```python
from build123d import *

# Parameters (mm, degrees)
SKETCH_1_R          = 6
EXTRUDE_1_DEPTH     = 1
SKETCH_2_R          = 4.075
SKETCH_2_R_2        = 3
EXTRUDE_2_DEPTH     = 3
CUT_EXTRUDE_START   = -3
SKETCH_3_R          = 3
CUT_EXTRUDE_1_DEPTH = 3
CHAMFER_1_SIZE      = 0.5


with BuildPart() as part:
    # 草图1 → 凸台-拉伸1 (new body)
    with BuildSketch(Plane(origin=(0, 0, 0), x_dir=(1, 0, 0), z_dir=(0, 1, 0))):
        with Locations(Location((-0.138701754, 0.180249091, 0), (0, 0, 270))):
            Circle(SKETCH_1_R)
    extrude(amount=EXTRUDE_1_DEPTH)

    # 草图2 → 凸台-拉伸2 (add)
    with BuildSketch(Plane(origin=(0, 1, 0), x_dir=(1, 0, 0), z_dir=(0, 1, 0))):
        with Locations(Location((-0.138701754, 0.180249091, 0), (0, 0, 270))):
            Circle(SKETCH_2_R)
        with Locations(Location((-0.138701754, 0.180249091, 0), (0, 0, 270))):
            Circle(SKETCH_2_R_2, mode=Mode.SUBTRACT)
    extrude(amount=EXTRUDE_2_DEPTH)

    # 草图3 → 切除-拉伸1 (cut)
    with BuildSketch(Plane(origin=(0, 1, 0), x_dir=(1, 0, 0), z_dir=(0, 1, 0)).offset(CUT_EXTRUDE_START)):
        with Locations(Location((-0.138701754, 0.180249091, 0), (0, 0, 270))):
            Circle(SKETCH_3_R)
    extrude(amount=CUT_EXTRUDE_1_DEPTH, mode=Mode.SUBTRACT)

    # 倒角1
    chamfer_1_edges = [part.edges().sort_by_distance(p)[0] for p in [
        (-0.138701754, 4, -4.255249091),
    ]]
    chamfer(chamfer_1_edges, length=CHAMFER_1_SIZE)


solid = part.part
```
Source: CAD feature listing. Evaluate the final solid. Frame: model axes, mm. Give positions to 0.01 mm unless a question says otherwise; leave off trailing zeros. Loops run counter-clockwise (first coordinate to the right, second up) from the corner with the lowest first, then second, coordinate; pieces in that order, holes last. Notation, with made-up numbers: M -27,51.5 L -12,51.5 A22 cw -12,58.5 Z; hole C -17,0.25 d10. An arc over 180 degrees is marked long. Put each result on its own line as item: value.
Q1. Mould query, pull axis Z, two halves, no side actions, for faces 1 (the flat face through (-1, 1, 4)), 2 (the cylindrical face through (-2.618, 2.232, -3.414)), 3 (the cylindrical face through (-1.29, 1.97, 2.59)). Classes: released by +Z, released by -Z, zero draft, split by the parting line, or undercut.
Response values:
face 1: zero draft
face 2: split by the parting line
face 3: undercut
Q2. Section B-B (x = 5). Return the cut outline in (y, z).
Response values:
outline: M 0,-3.28 L 1,-3.28 L 1,2.92 L 0,2.92 Z
Q3. Section C-C (z = 4.25). Return the cut outline in (x, y).
Response values:
outline: M -4.19,0 L 3.91,0 L 3.91,1 L -4.19,1 Z
Q4. Line query: probe 1 along Z at (x, y) = (-1.25, 2.9); probe 2 along Y at (x, z) = (0.75, -3.75); probe 3 along Z at (x, y) = (1.75, 0.2). Output: solid intervals per line, ascending. Write a range as [from, to].
Response values:
probe 1: z = [-4.1, -2.97], [2.61, 3.74]
probe 2: y = [0, 3.9]
probe 3: z = [-5.88, -2.51], [2.15, 5.51]
Q5. Pin query (flat end, axial travel): P1, Ø3, axis at x = -3, z = 4.5, coming from the +Y side; P2, Ø1, axis at y = 2, z = -2.5, coming from the +X side. Return the tip coordinate at first contact, or that it passes through.
Response values:
P1: stops at y = 3.59
P2: stops at x = 3.51
Q6. Section A-A (y = 0.55). Return the cut outline in (x, z), and give its area (3 significant figures).
Response values:
outline: C -0.14,-0.18 d12; hole C -0.14,-0.18 d6
area: 84.8 mm²
Q7. Section D-D (y = 2.7). Return the cut outline in (x, z) (3 decimals), and give its area (3 significant figures).
Response values:
outline: C -0.139,-0.18 d8.15; hole C -0.139,-0.18 d6
area: 23.9 mm²
